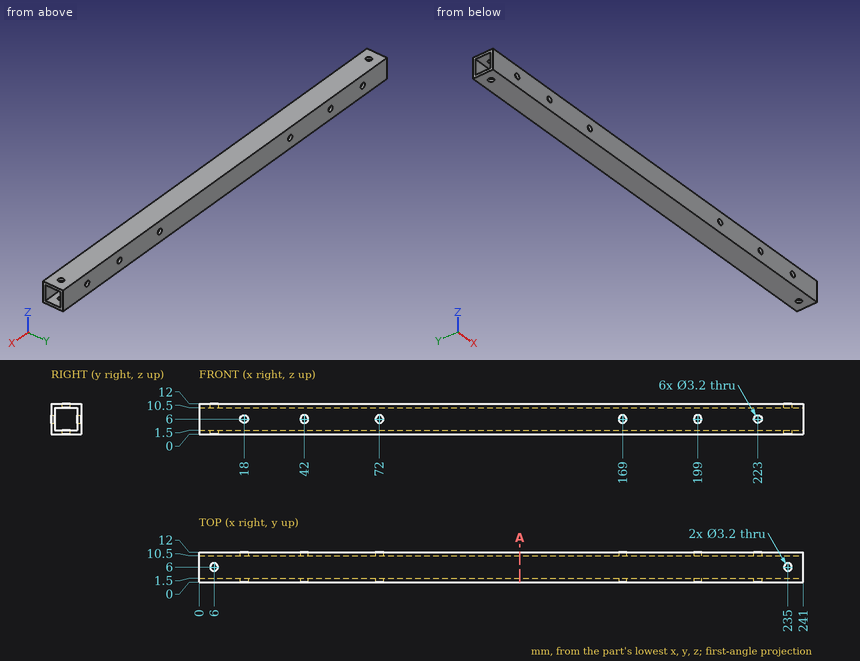
Design review of the part shown in the three views and the two pictorial views. Dimensions are in mm from the part's minimum x, y and z. Coordinates: 2 decimals unless noted, no trailing zeros. Order: outer loops, then holes, each group sorted by start corner. A loop starts at its lowest first (then second) coordinate and runs counter-clockwise, first axis right, second up.
Item 1: Take a section at A-A, the plane x = 128. Write out the cut boundary in (y, z).
Item 2: For line 1 (Y direction, x = 27, z = 6.25); line 2 (Z direction, x = 18, y = 0.4), list the stretches that pass through material, from the lowest coordinate up.
Item 3: For pin 1 Ø2.5 at (x, z) = (18, 6) entering from +Y, flat-tipped, find the tip position at first contact; note if it passes through.
The answers:
1. outline: (0, 0) - (12, 0) - (12, 12) - (0, 12) - close; hole (1.5, 1.5) - (10.5, 1.5) - (10.5, 10.5) - (1.5, 10.5) - close
2. line 1: y = 0 to 1.5, 10.5 to 12
2. line 2: z = 0 to 4.4, 7.6 to 12
3. pin 1: passes through
